Part model, mm, in its own coordinate system. Face numbers are marked on the shaded views. A direction names the side the tool comes from. Round coordinates to 2 decimals unless told otherwise and drop trailing zeros. Write each loop counter-clockwise with the first axis right and the second up, starting at its lowest first coordinate (ties: lowest second). Pieces come first, ordered by that corner, then holes.
from build123d import *

# Parameters (mm, degrees)
SKETCH3_W                                         = 141.6
SKETCH3_H                                         = 62.6
SKETCH3_W_2                                       = 137
SKETCH3_H_2                                       = 58
BOSS_EXTRUDE1_DEPTH                               = 10.5
SKETCH5_W                                         = 137
SKETCH5_H                                         = 58
BOSS_EXTRUDE2_DEPTH                               = 2
SKETCH6_R                                         = 3
BOSS_EXTRUDE3_DEPTH                               = 8.5
FILLET6_R                                         = 2
FILLET8_R                                         = 2
CHAMFER1_SIZE                                     = 1
SKETCH24_R                                        = 4.3
BOSS_EXTRUDE7_DEPTH                               = 8.5
FILLET21_R                                        = 2
FILLET22_R                                        = 2
FILLET20_R                                        = 4.3
CSK_FOR_4_FLAT_HEAD_SOCKET_CAP_SCREW1_D           = 3.4544
CSK_FOR_4_FLAT_HEAD_SOCKET_CAP_SCREW1_DEPTH       = 14
CSK_FOR_4_FLAT_HEAD_SOCKET_CAP_SCREW1_CSINK_D     = 6.723761
CSK_FOR_4_FLAT_HEAD_SOCKET_CAP_SCREW1_CSINK_ANGLE = 82
CSK_FOR_4_FLAT_HEAD_SOCKET_CAP_SCREW1_TIP         = 1.037806461
CHAMFER7_SIZE                                     = 1


# Some blends are built 0.0001 mm under size
with BuildPart() as part:
    # Sketch3 → Boss-Extrude1 (new body)
    with BuildSketch(Plane(origin=(0, 0, 0), x_dir=(1, 0, 0), z_dir=(0, 1, 0))):
        with Locations((-4.061766162, 3.105993834)):
            Rectangle(SKETCH3_W, SKETCH3_H)
        with Locations((-4.061766162, 3.105993834)):
            Rectangle(SKETCH3_W_2, SKETCH3_H_2, mode=Mode.SUBTRACT)
    extrude(amount=BOSS_EXTRUDE1_DEPTH)

    # Sketch5 → Boss-Extrude2 (add)
    with BuildSketch(Plane(origin=(0, 0, 0), x_dir=(1, 0, 0), z_dir=(0, 1, 0))):
        with Locations((-4.061766162, 3.105993834)):
            Rectangle(SKETCH5_W, SKETCH5_H)
    extrude(amount=BOSS_EXTRUDE2_DEPTH)

    # Sketch6 → Boss-Extrude3 (add)
    with BuildSketch(Plane(origin=(0, 2, 0), x_dir=(1, 0, 0), z_dir=(0, 1, 0))):
        with Locations(Location((-68.061766162, 27.605993834, 0), (0, 0, 270))):
            Circle(SKETCH6_R)
        with Locations(Location((-68.061766162, -21.394006166, 0), (0, 0, 270))):
            Circle(SKETCH6_R)
        with Locations(Location((-10.061766162, -21.394006166, 0), (0, 0, 270))):
            Circle(SKETCH6_R)
        with Locations(Location((-10.061766162, 27.605993834, 0), (0, 0, 270))):
            Circle(SKETCH6_R)
    extrude(amount=BOSS_EXTRUDE3_DEPTH)

    # Fillet6
    fillet6_edges = [part.edges().sort_by_distance(p)[0] for p in [
        (64.438233838, 6.25, -32.105993834),
    ]]
    fillet(fillet6_edges, radius=FILLET6_R)

    # Fillet8
    fillet8_edges = [part.edges().sort_by_distance(p)[0] for p in [
        (-72.561766162, 6.25, -32.105993834),
        (-72.561766162, 6.25, 25.894006166),
    ]]
    fillet(fillet8_edges, radius=FILLET8_R)

    # Chamfer1
    chamfer1_edges = [part.edges().sort_by_distance(p)[0] for p in [
        (-68.061766162, 2, -30.605993834),
        (-68.061766162, 2, 18.394006166),
        (-10.061766162, 2, 18.394006166),
        (-10.061766162, 2, -30.605993834),
    ]]
    chamfer(chamfer1_edges, length=CHAMFER1_SIZE)

    # Sketch24 → Boss-Extrude7 (add)
    with BuildSketch(Plane(origin=(0, 2, 0), x_dir=(1, 0, 0), z_dir=(0, 1, 0))):
        with Locations((62.438233838, -23.894006166)):
            Circle(SKETCH24_R)
        with Locations((62.438233838, 30.01834388)):
            Circle(SKETCH24_R)
    extrude(amount=BOSS_EXTRUDE7_DEPTH)

    # Fillet21
    fillet21_edges = [part.edges().sort_by_distance(p)[0] for p in [
        (58.631660576, 6.25, 25.894006166),
    ]]
    fillet(fillet21_edges, radius=FILLET21_R)

    # Fillet22
    fillet22_edges = [part.edges().sort_by_distance(p)[0] for p in [
        (64.438233838, 6.25, -26.211770618),
        (58.679016144, 6.25, -32.105993834),
        (64.438233838, 6.25, 20.087432904),
    ]]
    fillet(fillet22_edges, radius=FILLET22_R)

    # Fillet20
    fillet20_edges = [part.edges().sort_by_distance(p)[0] for p in [
        (-74.861766162, 5.25, -34.405993834),
        (66.738233838, 5.25, -34.405993834),
        (66.738233838, 5.25, 28.194006166),
        (-74.861766162, 5.25, 28.194006166),
    ]]
    fillet(fillet20_edges, radius=FILLET20_R - 0.0001)  # a hair under: the kernel refuses the full size

    # CSK for #4 Flat Head Socket Cap Screw1
    with Locations(Plane(origin=(0, 0, 0), x_dir=(-1, 0, 0), z_dir=(0, -1, 0))):
        with Locations((68.061766162, 27.605993834), (68.061766162, -21.394006166), (-62.438233838, 30.105993834), (-62.438233838, -23.894006166), (10.061766162, -21.394006166), (10.061766162, 27.605993834)):
            CounterSinkHole(CSK_FOR_4_FLAT_HEAD_SOCKET_CAP_SCREW1_D / 2, CSK_FOR_4_FLAT_HEAD_SOCKET_CAP_SCREW1_CSINK_D / 2, depth=CSK_FOR_4_FLAT_HEAD_SOCKET_CAP_SCREW1_DEPTH, counter_sink_angle=CSK_FOR_4_FLAT_HEAD_SOCKET_CAP_SCREW1_CSINK_ANGLE)
            with Locations((0, 0, -(CSK_FOR_4_FLAT_HEAD_SOCKET_CAP_SCREW1_DEPTH + CSK_FOR_4_FLAT_HEAD_SOCKET_CAP_SCREW1_TIP / 2))):  # 118° drill point
                Cone(0, CSK_FOR_4_FLAT_HEAD_SOCKET_CAP_SCREW1_D / 2, CSK_FOR_4_FLAT_HEAD_SOCKET_CAP_SCREW1_TIP, mode=Mode.SUBTRACT)

    # Chamfer7
    # the kernel refuses this chamfer: 1 mm, written as the material it takes off along each edge
    with BuildSketch(Plane(origin=(62.438333838, 0, -34.405993834), x_dir=(0, -0.027495876610586292, 0.9996219169112968), z_dir=(-1, 0, 0)), Plane(origin=(-70.561866162, 0, 28.194006166), x_dir=(0, -0.02749587661058639, -0.9996219169112968), z_dir=(1, 0, 0))) as chamfer7_piece_1:
        Polygon((CHAMFER7_SIZE * 0.999621916911, CHAMFER7_SIZE * 0.0274958766106), (-CHAMFER7_SIZE * 0.0274958766106, CHAMFER7_SIZE * 0.999621916911), (0, 0), align=None)
    extrude(amount=133.0002, mode=Mode.SUBTRACT)
    with BuildSketch(Plane(origin=(-74.861766162, 0, -30.106093834), x_dir=(0.9996219169112968, -0.027495876610586483, 0), z_dir=(0, 0, 1)), Plane(origin=(66.738233838, 0, 23.894106166), x_dir=(-0.9996219169112968, -0.027495876610586483, 0), z_dir=(0, 0, -1))) as chamfer7_piece_2:
        Polygon((CHAMFER7_SIZE * 0.999621916911, CHAMFER7_SIZE * 0.0274958766106), (-CHAMFER7_SIZE * 0.0274958766106, CHAMFER7_SIZE * 0.999621916911), (0, 0), align=None)
    extrude(amount=54.0002, mode=Mode.SUBTRACT)
    with BuildSketch(Plane(origin=(62.438333838, 0, 23.894106166), x_dir=(0, 0, 1), z_dir=(-1, 0, 0))) as chamfer7_piece_3:
        Polygon((4.2999 - CHAMFER7_SIZE, 0), (4.2999, CHAMFER7_SIZE), (4.2999, 0), align=None)
    revolve(axis=Axis((62.438333838, 0, 23.894106166), (0, 1, 0)), revolution_arc=90, mode=Mode.SUBTRACT)
    with BuildSketch(Plane(origin=(-70.561866162, 0, 23.894106166), x_dir=(0, 0, 1), z_dir=(1, 0, 0))) as chamfer7_piece_4:
        Polygon((4.2999 - CHAMFER7_SIZE, 0), (4.2999, -CHAMFER7_SIZE), (4.2999, 0), align=None)
    revolve(axis=Axis((-70.561866162, 0, 23.894106166), (0, -1, 0)), revolution_arc=90, mode=Mode.SUBTRACT)
    with BuildSketch(Plane(origin=(-70.561866162, 0, -30.106093834), x_dir=(0, 0, -1), z_dir=(1, 0, 0))) as chamfer7_piece_5:
        Polygon((4.2999 - CHAMFER7_SIZE, 0), (4.2999, CHAMFER7_SIZE), (4.2999, 0), align=None)
    revolve(axis=Axis((-70.561866162, 0, -30.106093834), (0, 1, 0)), revolution_arc=90, mode=Mode.SUBTRACT)
    with BuildSketch(Plane(origin=(62.438333838, 0, -30.106093834), x_dir=(1, 0, 0), z_dir=(0, 0, 1))) as chamfer7_piece_6:
        Polygon((4.2999 - CHAMFER7_SIZE, 0), (4.2999, CHAMFER7_SIZE), (4.2999, 0), align=None)
    revolve(axis=Axis((62.438333838, 0, -30.106093834), (0, 1, 0)), revolution_arc=90, mode=Mode.SUBTRACT)


solid = part.part
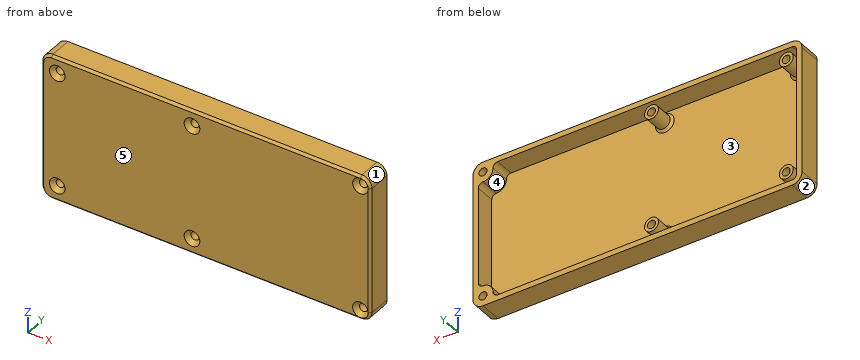
Q1. Tool access for the marked faces 4 and 5: list every direction of +Z, -Z, +X, -X, +Y, -Y with a clear straight run to the whole face (end or side of a thin tool).
Q2. Saw through at B-B, the plane y = 5. Give the number of separate pieces and of enclosed holes in the cut face, and give its area (3 significant figures).
Q3. Saw through at A-A, the plane x = 26. Write the cut outline in (y, z).
Q4. Saw through at C-C, the plane z = -11.5. Write the cut outline in (x, y).
Q5. Two-plate mould, pull along X, no slides. Class the marked faces 1, 2 and 3: released by +X, released by -X, zero draft, split by the parting line, or undercut.
Q6. Wall check: line 1 (Z direction, x = 46, y = 3.25); line 2 (X direction, y = 7, z = -21); line 3 (X direction, y = 8.75, z = 22). Give the ranges that are in metal, low to high.
Q7. Drop flat-ended pins along their axis: P1, Ø3, axis at x = -10.5, z = -9, coming from the +Y side; P2, Ø4, axis at x = -10.06, z = -27.61, coming from the -Y side; P3, Ø5.5, axis at x = 62.44, z = -30.11, coming from the -Y side. Give the stop position or say it passes through.
Computed:
1. face 4: +Y
1. face 5: +Z, -Z, +X, -X, -Y
2. separate pieces: 5
2. enclosed holes: 7
2. area: 1,040 mm2
3. outline: (0, -33.41) - (1, -34.41) - (10.5, -34.41) - (10.5, -32.11) - (2, -32.11) - (2, 25.89) - (10.5, 25.89) - (10.5, 28.19) - (1, 28.19) - (0, 27.19) - close
4. outline: (-74.86, 1) - (-73.86, 0) - (65.74, 0) - (66.74, 1) - (66.74, 10.5) - (64.44, 10.5) - (64.44, 2) - (-72.56, 2) - (-72.56, 10.5) - (-74.86, 10.5) - close
5. face 1: released by +X
5. face 2: released by -X
5. face 3: undercut
6. line 1: z = -34.41 to -32.11, 25.89 to 28.19
6. line 2: x = -74.86 to -72.56, 64.44 to 66.74
6. line 3: x = -74.86 to -72.56, -71 to -69.68, -66.44 to -65.12, -13 to -11.68, -8.44 to -7.12, 58.58 to 66.74
7. P1: stops at y = 2
7. P2: stops at y = 1.56
7. P3: stops at y = 0.7
